from build123d import *

# Parameters (mm, degrees)
SKETCH1_R           = 2.5
SKETCH1_R_2         = 1
BOSS_EXTRUDE2_DEPTH = 2.1
SKETCH2_R           = 1
BOSS_EXTRUDE3_DEPTH = 1
SKETCH4_R           = 1
CUT_EXTRUDE13_DEPTH = 2
SKETCH6_OUTSIDE_W   = 8.99
SKETCH6_OUTSIDE_H   = 8.99
SKETCH6_OUTSIDE_R   = 2.5
CUT_EXTRUDE14_DEPTH = 8.842193571


with BuildPart() as part:
    # Sketch1 → Boss-Extrude2 (new body)
    with BuildSketch(Plane(origin=(0, 0, 0), x_dir=(1, 0, 0), z_dir=(0, 1, 0))):
        with Locations(Location((0, 0, 0), (0, 0, 270))):
            Circle(SKETCH1_R)
        with Locations(Location((0, 0, 0), (0, 0, 270))):
            Circle(SKETCH1_R_2, mode=Mode.SUBTRACT)
    extrude(amount=BOSS_EXTRUDE2_DEPTH)

    # Sketch2 → Boss-Extrude3 (add, symmetric)
    with BuildSketch(Plane.XY):
        with BuildLine():
            Line((2.5, 4.5), (2.5, 0))
            Line((2.5, 0), (-2.5, 0))
            Line((-2.5, 0), (-2.5, 4.5))
            ThreePointArc((-2.5, 4.5), (0, 7), (2.5, 4.5))
        make_face()
        with Locations((0, 4.5)):
            Circle(SKETCH2_R, mode=Mode.SUBTRACT)
    extrude(amount=BOSS_EXTRUDE3_DEPTH, both=True)

    # Sketch4 → Cut-Extrude13 (cut)
    with BuildSketch(Plane.XZ):
        with Locations(Location((0, 0, 0), (0, 0, 270))):
            Circle(SKETCH4_R)
    extrude(amount=-CUT_EXTRUDE13_DEPTH, mode=Mode.SUBTRACT)

    # Sketch6 outside → Cut-Extrude14 (cut, through all)
    with BuildSketch(Plane.XZ):
        Rectangle(SKETCH6_OUTSIDE_W, SKETCH6_OUTSIDE_H)
        with Locations(Location((0, 0, 0), (0, 0, 336.421821522))):
            Circle(SKETCH6_OUTSIDE_R, mode=Mode.SUBTRACT)
    extrude(amount=-CUT_EXTRUDE14_DEPTH, mode=Mode.SUBTRACT)


solid = part.part
Input: part model. Units: mm. Frame: model coordinates. A direction names the side the tool comes from. Give positions to 0.01 mm unless a question says otherwise; leave off trailing zeros. Loops run counter-clockwise (first coordinate to the right, second up) from the corner with the lowest first, then second, coordinate; pieces in that order, holes last. Notation, with made-up numbers: (22.5, -1) -> (79.5, -1) arc R21 cw to (79.5, 21) -> close; hole circle Ø8 at (-34.75, -0.5). An arc over 180 degrees is marked (long way). Answer as a JSON object with one key per item and string values. Group by question number.
Item 1: Cut plane B-B, the plane z = 0. Return the cut outline in (x, y), and give its area (3 significant figures).
Item 2: Cut plane C-C, the plane y = 1.75. Return the cut outline in (x, z), and give its area (3 significant figures).
Item 3: Cut plane A-A, the plane x = 0. Return the cut outline in (y, z).
Item 4: Pin query (flat end, axial travel): P1, Ø2.5, axis at x = -0.5, y = 5.5, coming from the -Z side; P2, Ø1, axis at x = -1.5, y = 5.5, coming from the +Z side; P3, Ø1.6, axis at x = 1, z = -2, coming from the +Y side; P4, Ø1.6, axis at x = 0, y = 4.5, coming from the +Z side. Return the tip coordinate at first contact, or that it passes through.
Item 5: Pull-direction query (X, two-part tool) for faces 4 (the cylindrical face through (0.17, 1.489, -2.494)), 5 (the flat face through (0, 2.1, -2)), 6 (the flat face through (0, 2, 0)); classes: released by +X, released by -X, zero draft, split by the parting line, or undercut.
Item 6: Cut plane D-D, the plane x = -2.1. Return the cut outline in (y, z), and give its area (3 significant figures).
Item 7: Reachability of faces 1 (the flat face through (0, 3, -1)), 2 (the flat face through (0, 3, 1)), 3 (the cylindrical face through (-1, 1, 0)) from +Z, -Z, +X, -X, +Y, -Y: full face, straight path, thin tool, end or side. Return the list, or none.
Item 8: Line query: probe 1 along X at (y, z) = (0.5, 0); probe 2 along Y at (x, z) = (0, -0.55); probe 3 along Z at (x, y) = (1.4, 5.5). Output: solid intervals per line, ascending.
Checks:
{
 "1": {"outline": "(-2.5, 0) -> (-1, 0) -> (-1, 2) -> (1, 2) -> (1, 0) -> (2.5, 0) -> (2.5, 4.5) arc R2.5 ccw to (-2.5, 4.5) -> close; hole circle Ø2 at (0, 4.5)", "area": "25.2 mm²"},
 "2": {"outline": "circle Ø5 at (0, 0); hole circle Ø2 at (0, 0)", "area": "16.5 mm²"},
 "3": {"outline": "(0, -2.5) -> (2.1, -2.5) -> (2.1, -1) -> (3.5, -1) -> (3.5, 1) -> (2.1, 1) -> (2.1, 2.5) -> (0, 2.5) -> (0, 1) -> (2, 1) -> (2, -1) -> (0, -1) -> close; (5.5, -1) -> (7, -1) -> (7, 1) -> (5.5, 1) -> close"},
 "4": {"P1": "stops at z = -1", "P2": "stops at z = 1", "P3": "stops at y = 2.1", "P4": "passes through"},
 "5": {"face 4": "split by the parting line", "face 5": "zero draft", "face 6": "undercut"},
 "6": {"outline": "(0, -1.36) -> (2.1, -1.36) -> (2.1, -1) -> (5.86, -1) -> (5.86, 1) -> (2.1, 1) -> (2.1, 1.36) -> (0, 1.36) -> close", "area": "13.2 mm²"},
 "7": {"face 1": "-Z, +X, -X, +Y", "face 2": "+Z, +X, -X, +Y", "face 3": "-Y"},
 "8": {"probe 1": "x = -2.5 to -1, 1 to 2.5", "probe 2": "y = 2 to 3.5, 5.5 to 7", "probe 3": "z = -1 to 1"}
}
